Can you work these out from the model? Positions are in its coordinate system, mm. Face numbers are marked on the shaded views. A direction names the side the tool comes from. Give positions to 0.01 mm unless a question says otherwise; leave off trailing zeros. Order: outer loops, then holes, each group sorted by start corner. A loop starts at its lowest first (then second) coordinate and runs counter-clockwise, first axis right, second up. Notation, with made-up numbers: M 21,6 L 37,6 A18 cw 37,20 Z; hole C 61.5,-34 d6. An arc over 180 degrees is marked long. One line per question, with ' | ' between items. Start each with the question number.
1) If we section it at B-B, the plane y = -10: Please give me the cut outline in (x, z), plus the area to 3 significant figures.
2) Please list where these lines run through material, in increasing order: line 1 along Y through (x, z) = (6, 27); line 2 along X through (y, z) = (5.5, 22); line 3 along Z through (x, y) = (-24, -9.5). Write a range as [from, to].
3) If we section it at A-A, the plane x = 6.5: Please give me the cut outline in (y, z), plus the area to 3 significant figures.
4) I'm going to push flat-ended pins straight in: pin 1 Ø1.2 at (x, z) = (1.5, 0.5) entering from -Y; pin 2 Ø0.5 at (x, z) = (0, 1) entering from +Y; pin 3 Ø8.5 at (y, z) = (7, 25) entering from +X. Where does each tip first touch, or does it pass through?
5) If we section it at C-C, the plane z = 13: Please give me the cut outline in (x, y), plus the area to 3 significant figures.
6) For the marked faces 4 and 5, which set-ups out of +Z, -Z, +X, -X, +Y, -Y let a thin tool reach every point of the face, with its end or its side?
7) If we section it at D-D, the plane x = -18.5: Please give me the cut outline in (y, z), plus the area to 3 significant figures.
8) Thinking about a two-plate mould opening in Y: for the marked faces 1, 2 and 3, which applies, +Y half, -Y half, draft (parallel to the pull), parting line (faces both ways), or undercut?
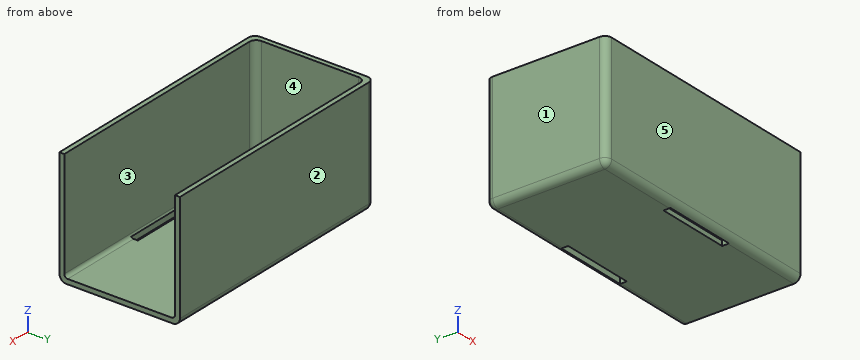
```python
from build123d import *

# Parameters (mm, degrees)
F0_W         = 74.44
F0_H         = 35.44
F1_DEPTH     = 34
F2_T         = -1.44
F3_DEPTH     = 1.44
F4_R         = 2
F5_R         = 2
F6_W         = 22
F6_H         = 2
F7_DEPTH     = 1.441
F8_T1_DEPTH  = 28.56
F8_T6_DEPTH  = 69.56
F8_T12_DEPTH = 69.56
F8_T18_DEPTH = 69.56
F8_T25_DEPTH = 69.56
F8_T31_DEPTH = 69.56
F8_T35_ANGLE = 90
F8_T37_ANGLE = 90
F8_T41_DEPTH = 69.56
F8_T47_DEPTH = 69.56
F8_T53_DEPTH = 69.56
F8_T60_DEPTH = 69.56
F8_T66_DEPTH = 69.56


# Not quite as in the source:
# - a fillet or chamfer that OpenCascade refuses, or shapes differently, is made with other operations: its cross-section is extruded or revolved along the edge and cut away or added


with BuildPart() as f1:
    # F0 (on Top) → F1 (new body)
    with BuildSketch(Plane.XY):
        Rectangle(F0_W, F0_H)
    extrude(amount=F1_DEPTH)

    # F2
    f2_openings = [f1.faces().sort_by_distance(p)[0] for p in [
        (0, 0, 34),
    ]]
    offset(amount=F2_T, openings=f2_openings)

    # F3 (cut): a face of the model
    f3_faces = [f1.faces().sort_by_distance(p)[0] for p in [
        (37.22, 0, 17),
    ]]
    extrude(f3_faces, amount=-F3_DEPTH, mode=Mode.SUBTRACT)

    # F4
    f4_edges = [f1.edges().sort_by_distance(p)[0] for p in [
        (-35.78, -16.28, 17.72),
        (-35.78, 16.28, 17.72),
        (-37.22, 17.72, 17),
        (-37.22, -17.72, 17),
    ]]
    fillet(f4_edges, radius=F4_R)

    # F5
    f5_edges = [f1.edges().sort_by_distance(p)[0] for p in [
        (-37.22, 0, 0),
        (0.28, -17.72, 0),
        (0.28, 17.72, 0),
    ]]
    fillet(f5_edges, radius=F5_R)

    # F6 (on face) → F7 (cut, through all)
    with BuildSketch(Plane.XY.offset(1.44)):
        with Locations((0, 15.03)):
            Rectangle(F6_W, F6_H)
        with Locations((0, -15.03)):
            Rectangle(F6_W, F6_H)
    extrude(amount=-F7_DEPTH, mode=Mode.SUBTRACT)

    # F8: fillet of radius 1 on 1 edges, made by hand

    # F8_s2 → F8_t1 (join)
    with BuildSketch(Plane.XZ.offset(-14.28)):
        with BuildLine():
            ThreePointArc((-35.78, 2.44), (-35.4871067812, 1.7328932188), (-34.78, 1.44))
            Line((-34.78, 1.44), (-35.78, 1.44))
            Line((-35.78, 1.44), (-35.78, 2.44))
        make_face()
    extrude(amount=F8_T1_DEPTH)


with BuildPart() as f8_tool4:
    # F8_s5 → F8_t6 (new body)
    with BuildSketch(Plane.YZ.offset(-33.78)):
        with BuildLine():
            ThreePointArc((-16.28, 2.44), (-15.9871067812, 1.7328932188), (-15.28, 1.44))
            Line((-15.28, 1.44), (-16.28, 1.44))
            Line((-16.28, 1.44), (-16.28, 2.44))
        make_face()
    extrude(amount=F8_T6_DEPTH)

    split(bisect_by=Plane.YZ.offset(-11), keep=Keep.BOTTOM)

    split(bisect_by=Plane.XZ.offset(16.03), keep=Keep.TOP)


with BuildPart() as f1_1:
    add(f1.part)

    # F8_t3: union F8_tool4
    add(f8_tool4.part)


with BuildPart() as f8_tool10:
    # F8_s11 → F8_t12 (new body)
    with BuildSketch(Plane.YZ.offset(-33.78)):
        with BuildLine():
            ThreePointArc((-16.28, 2.44), (-15.9871067812, 1.7328932188), (-15.28, 1.44))
            Line((-15.28, 1.44), (-16.28, 1.44))
            Line((-16.28, 1.44), (-16.28, 2.44))
        make_face()
    extrude(amount=F8_T12_DEPTH)

    split(bisect_by=Plane.YZ.offset(-11), keep=Keep.BOTTOM)

    split(bisect_by=Plane.XZ.offset(16.03), keep=Keep.BOTTOM)


with BuildPart() as f1_2:
    add(f1_1.part)

    # F8_t9: union F8_tool10
    add(f8_tool10.part)


with BuildPart() as f8_tool16:
    # F8_s17 → F8_t18 (new body)
    with BuildSketch(Plane.YZ.offset(-33.78)):
        with BuildLine():
            ThreePointArc((-16.28, 2.44), (-15.9871067812, 1.7328932188), (-15.28, 1.44))
            Line((-15.28, 1.44), (-16.28, 1.44))
            Line((-16.28, 1.44), (-16.28, 2.44))
        make_face()
    extrude(amount=F8_T18_DEPTH)

    split(bisect_by=Plane.YZ.offset(-11), keep=Keep.TOP)

    split(bisect_by=Plane.XZ.offset(16.03), keep=Keep.TOP)

    split(bisect_by=Plane.YZ.offset(11), keep=Keep.BOTTOM)


with BuildPart() as f1_3:
    add(f1_2.part)

    # F8_t15: union F8_tool16
    add(f8_tool16.part)


with BuildPart() as f8_tool23:
    # F8_s24 → F8_t25 (new body)
    with BuildSketch(Plane.YZ.offset(-33.78)):
        with BuildLine():
            ThreePointArc((-16.28, 2.44), (-15.9871067812, 1.7328932188), (-15.28, 1.44))
            Line((-15.28, 1.44), (-16.28, 1.44))
            Line((-16.28, 1.44), (-16.28, 2.44))
        make_face()
    extrude(amount=F8_T25_DEPTH)

    split(bisect_by=Plane.XZ.offset(16.03), keep=Keep.TOP)

    split(bisect_by=Plane.YZ.offset(11), keep=Keep.TOP)


with BuildPart() as f1_4:
    add(f1_3.part)

    # F8_t22: union F8_tool23
    add(f8_tool23.part)


with BuildPart() as f8_tool29:
    # F8_s30 → F8_t31 (new body)
    with BuildSketch(Plane.YZ.offset(-33.78)):
        with BuildLine():
            ThreePointArc((-16.28, 2.44), (-15.9871067812, 1.7328932188), (-15.28, 1.44))
            Line((-15.28, 1.44), (-16.28, 1.44))
            Line((-16.28, 1.44), (-16.28, 2.44))
        make_face()
    extrude(amount=F8_T31_DEPTH)

    split(bisect_by=Plane.XZ.offset(16.03), keep=Keep.BOTTOM)

    split(bisect_by=Plane.YZ.offset(11), keep=Keep.TOP)


with BuildPart() as f1_5:
    add(f1_4.part)

    # F8_t28: union F8_tool29
    add(f8_tool29.part)

    # F8_s34 → F8_t35 (revolve)
    with BuildSketch(Plane.XZ.offset(14.28)):
        with BuildLine():
            ThreePointArc((-35.78, 2.44), (-35.4871067812, 1.7328932188), (-34.78, 1.44))
            Line((-34.78, 1.44), (-35.78, 1.44))
            Line((-35.78, 1.44), (-35.78, 2.44))
        make_face()
    revolve(axis=Axis((-33.78, -14.28, 1.44), (0, 0, 1)), revolution_arc=F8_T35_ANGLE)

    # F8_s36 → F8_t37 (revolve)
    with BuildSketch(Plane.YZ.offset(-33.78)):
        with BuildLine():
            ThreePointArc((16.28, 2.44), (15.9871067812, 1.7328932188), (15.28, 1.44))
            Line((15.28, 1.44), (16.28, 1.44))
            Line((16.28, 1.44), (16.28, 2.44))
        make_face()
    revolve(axis=Axis((-33.78, 14.28, 1.44), (0, 0, 1)), revolution_arc=F8_T37_ANGLE)


with BuildPart() as f8_tool39:
    # F8_s40 → F8_t41 (new body)
    with BuildSketch(Plane.YZ.offset(35.78)):
        with BuildLine():
            ThreePointArc((16.28, 2.44), (15.9871067812, 1.7328932188), (15.28, 1.44))
            Line((15.28, 1.44), (16.28, 1.44))
            Line((16.28, 1.44), (16.28, 2.44))
        make_face()
    extrude(amount=-F8_T41_DEPTH)

    split(bisect_by=Plane.YZ.offset(11), keep=Keep.TOP)

    split(bisect_by=Plane.XZ.offset(-16.03), keep=Keep.BOTTOM)


with BuildPart() as f1_6:
    add(f1_5.part)

    # F8_t38: union F8_tool39
    add(f8_tool39.part)


with BuildPart() as f8_tool45:
    # F8_s46 → F8_t47 (new body)
    with BuildSketch(Plane.YZ.offset(35.78)):
        with BuildLine():
            ThreePointArc((16.28, 2.44), (15.9871067812, 1.7328932188), (15.28, 1.44))
            Line((15.28, 1.44), (16.28, 1.44))
            Line((16.28, 1.44), (16.28, 2.44))
        make_face()
    extrude(amount=-F8_T47_DEPTH)

    split(bisect_by=Plane.YZ.offset(11), keep=Keep.TOP)

    split(bisect_by=Plane.XZ.offset(-16.03), keep=Keep.TOP)


with BuildPart() as f1_7:
    add(f1_6.part)

    # F8_t44: union F8_tool45
    add(f8_tool45.part)


with BuildPart() as f8_tool51:
    # F8_s52 → F8_t53 (new body)
    with BuildSketch(Plane.YZ.offset(35.78)):
        with BuildLine():
            ThreePointArc((16.28, 2.44), (15.9871067812, 1.7328932188), (15.28, 1.44))
            Line((15.28, 1.44), (16.28, 1.44))
            Line((16.28, 1.44), (16.28, 2.44))
        make_face()
    extrude(amount=-F8_T53_DEPTH)

    split(bisect_by=Plane.YZ.offset(11), keep=Keep.BOTTOM)

    split(bisect_by=Plane.XZ.offset(-16.03), keep=Keep.BOTTOM)

    split(bisect_by=Plane.YZ.offset(-11), keep=Keep.TOP)


with BuildPart() as f1_8:
    add(f1_7.part)

    # F8_t50: union F8_tool51
    add(f8_tool51.part)


with BuildPart() as f8_tool58:
    # F8_s59 → F8_t60 (new body)
    with BuildSketch(Plane.YZ.offset(35.78)):
        with BuildLine():
            ThreePointArc((16.28, 2.44), (15.9871067812, 1.7328932188), (15.28, 1.44))
            Line((15.28, 1.44), (16.28, 1.44))
            Line((16.28, 1.44), (16.28, 2.44))
        make_face()
    extrude(amount=-F8_T60_DEPTH)

    split(bisect_by=Plane.XZ.offset(-16.03), keep=Keep.BOTTOM)

    split(bisect_by=Plane.YZ.offset(-11), keep=Keep.BOTTOM)


with BuildPart() as f1_9:
    add(f1_8.part)

    # F8_t57: union F8_tool58
    add(f8_tool58.part)


with BuildPart() as f8_tool64:
    # F8_s65 → F8_t66 (new body)
    with BuildSketch(Plane.YZ.offset(35.78)):
        with BuildLine():
            ThreePointArc((16.28, 2.44), (15.9871067812, 1.7328932188), (15.28, 1.44))
            Line((15.28, 1.44), (16.28, 1.44))
            Line((16.28, 1.44), (16.28, 2.44))
        make_face()
    extrude(amount=-F8_T66_DEPTH)

    split(bisect_by=Plane.XZ.offset(-16.03), keep=Keep.TOP)

    split(bisect_by=Plane.YZ.offset(-11), keep=Keep.BOTTOM)


with BuildPart() as f1_10:
    add(f1_9.part)

    # F8_t63: union F8_tool64
    add(f8_tool64.part)


solid = f1_10.part
```
Results found:
1) outline: M -37.22,2 A2 ccw -35.22,0 L 35.78,0 L 35.78,1.44 L -34.78,1.44 A1 cw -35.78,2.44 L -35.78,34 L -37.22,34 Z | area: 151 mm²
2) line 1: y = [-17.72, -16.28], [16.28, 17.72] | line 2: x = [-37.22, -35.78] | line 3: z = [0, 1.44]
3) outline: M -17.72,2 A2 ccw -16.03,0.02 L -16.03,1.78 A1 cw -16.28,2.44 L -16.28,34 L -17.72,34 Z; M -14.03,0 L 14.03,0 L 14.03,1.44 L -14.03,1.44 Z; M 16.03,0.02 A2 ccw 17.72,2 L 17.72,34 L 16.28,34 L 16.28,2.44 A1 cw 16.03,1.78 Z | area: 138 mm²
4) pin 1: stops at y = -17.51 | pin 2: stops at y = 17.57 | pin 3: stops at x = -35.78
5) outline: M -37.22,-15.72 A2 ccw -35.22,-17.72 L 35.78,-17.72 L 35.78,-16.28 L -33.78,-16.28 A2 cw -35.78,-14.28 L -35.78,14.28 A2 cw -33.78,16.28 L 35.78,16.28 L 35.78,17.72 L -35.22,17.72 A2 ccw -37.22,15.72 Z | area: 257 mm²
6) face 4: +Z, +X | face 5: +Z, -Z, +X, -X, -Y
7) outline: M -17.72,2 A2 ccw -15.72,0 L 15.72,0 A2 ccw 17.72,2 L 17.72,34 L 16.28,34 L 16.28,2.44 A1 cw 15.28,1.44 L -15.28,1.44 A1 cw -16.28,2.44 L -16.28,34 L -17.72,34 Z | area: 144 mm²
8) face 1: draft | face 2: +Y half | face 3: undercut
